from build123d import *

# Parameters (mm, degrees)
SKETCH1_W           = 12.5
SKETCH1_H           = 25
SKETCH1_W_2         = 10.1
SKETCH1_H_2         = 22.6
BOSS_EXTRUDE1_DEPTH = 400
SKETCH3_R           = 5
SKETCH3_R_2         = 2
CUT_EXTRUDE1_DEPTH  = 20


with BuildPart() as part:
    # Sketch1 → Boss-Extrude1 (new body)
    with BuildSketch(Plane(origin=(0, 0, 0), x_dir=(0, 0, -1), z_dir=(1, 0, 0))):
        Rectangle(SKETCH1_W, SKETCH1_H)
        Rectangle(SKETCH1_W_2, SKETCH1_H_2, mode=Mode.SUBTRACT)
    extrude(amount=BOSS_EXTRUDE1_DEPTH)

    # Sketch3 → Cut-Extrude1 (cut)
    with BuildSketch(Plane(origin=(0, 0, -6.25), x_dir=(-1, 0, 0), z_dir=(0, 0, -1))):
        with Locations((-200, 0)):
            Circle(SKETCH3_R)
        with Locations((-188, 0)):
            Circle(SKETCH3_R_2)
        with Locations((-212, 0)):
            Circle(SKETCH3_R_2)
    extrude(amount=-CUT_EXTRUDE1_DEPTH, mode=Mode.SUBTRACT)


solid = part.part
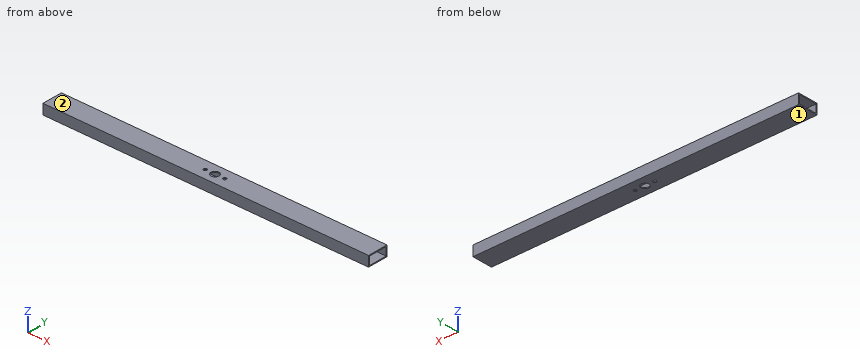
For this review, take the finished solid that the model builds, in its own axes (mm). Face numbers are marked on the shaded views. Coordinates: 2 decimals unless noted, no trailing zeros. Order: outer loops, then holes, each group sorted by start corner. A loop starts at its lowest first (then second) coordinate and runs counter-clockwise, first axis right, second up. Notation, with made-up numbers: (55, 41.5) - (87, 41.5) arc R27 cw to (87, 63.5) - close; hole circle Ø10 at (3.5, 35.25). An arc over 180 degrees is marked (long way). Answer as CSV lines item,"result". Start each with the question number.
1) Add section B-B (z = -0.75). State the section outline as (x, y) points.
2) Add section C-C (x = 148.5). State the section outline as (y, z) points.
3) Add section A-A (x = 200). State the section outline as (y, z) points.
4) Draft analysis for pull direction Z (two halves, no side actions). For the marked faces 1 and 2, state which applies: +Z half, -Z half, draft (parallel to the pull), parting line (faces both ways), or undercut.
5) To check wall thickness, follow line 1 along Z through (x, y) = (160, -3.75); line 2 along Y through (x, z) = (212, -5.7). State the ranges of each line that lie inside material, in increasing order. Write a range as [from, to].
Result:
1,outline,"(0, -12.5) - (400, -12.5) - (400, -11.3) - (0, -11.3) - close; (0, 11.3) - (400, 11.3) - (400, 12.5) - (0, 12.5) - close"
2,outline,"(-12.5, -6.25) - (12.5, -6.25) - (12.5, 6.25) - (-12.5, 6.25) - close; hole (-11.3, -5.05) - (11.3, -5.05) - (11.3, 5.05) - (-11.3, 5.05) - close"
3,outline,"(-12.5, -6.25) - (-5, -6.25) - (-5, -5.05) - (-11.3, -5.05) - (-11.3, 5.05) - (-5, 5.05) - (-5, 6.25) - (-12.5, 6.25) - close; (5, -6.25) - (12.5, -6.25) - (12.5, 6.25) - (5, 6.25) - (5, 5.05) - (11.3, 5.05) - (11.3, -5.05) - (5, -5.05) - close"
4,face 1,"-Z half"
4,face 2,"+Z half"
5,line 1,"[-6.25, -5.05], [5.05, 6.25]"
5,line 2,"[-12.5, -2], [2, 12.5]"
